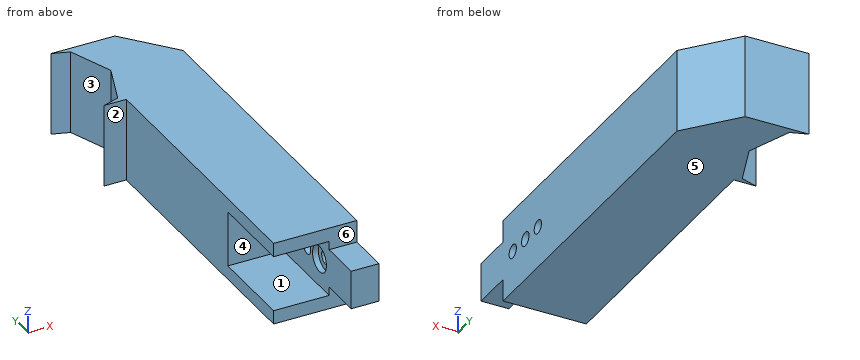
Autodesk Inventor part; units mm, degrees
ref_plane "YZ Plane" through (0, 0, 0) normal (1, 0, 0) x (0, 1, 0)
ref_plane "XZ Plane" through (0, 0, 0) normal (0, 1, 0) x (-1, 0, 0)
ref_plane "XY Plane" through (0, 0, 0) normal (0, 0, 1) x (1, 0, 0)
sketch "Sketch1" plane through (0, 0, 0) normal (0, 0, 1) x (1, 0, 0)
  line L0 (0, 0) -> (25, 0)
  line L1 (25, 0) -> (25, 40)
  line L2 (25, 40) -> (0, 40)
  line L3 (0, 40) -> (0, 0)
  dimension "d1" = 25
  dimension "d2" = 40
  dimension "d3" = 25
extrude "Extrusion1" add sketch "Sketch1" against normal blind 30
sketch "Sketch2" plane through (25, 0, 0) normal (1, 0, 0) x (0, 0, -1)
  line L0 (0, 0) -> (30, 0)
  circle A0 centre (15, 6.56) radius 2.46
extrude "Extrusion2" cut sketch "Sketch2" against normal blind 30
sketch "Sketch3" plane through (0, 0, 0) normal (-1, 0, 0) x (0, 0, 1)
  line L0 (0, 0) -> (-30, 0)
  line L1 (-25.05, 0) -> (-4.95, 0)
  line L2 (-4.95, 0) -> (-4.95, 33.12)
  line L3 (-4.95, 33.12) -> (-25.05, 33.12)
  line L4 (-25.05, 33.12) -> (-25.05, 0)
  dimension "d11" = 20.1
extrude "Extrusion3" cut sketch "Sketch3" against normal blind 20
sketch "Sketch4" plane through (0, 0, 0) normal (0, -1, 0) x (1, 0, 0)
  line L0 (20, -4.95) -> (20, -25.05)
  line L1 (20, -15) -> (25, -15)
  line L2 (25, 0) -> (25, -30)
  line L3 (20, -8.025) -> (25, -8.025)
  line L4 (25, -8.025) -> (25, -21.975)
  line L5 (25, -21.975) -> (20, -21.975)
  line L6 (20, -21.975) -> (20, -8.025)
  line L7 (20, -8.025) -> (25, -21.975) construction
  line L8 (25, -8.025) -> (20, -21.975) construction
  line L9 (25, -12.54) -> (25, -17.46)
  point P0 (0, 0)
  point P1 (22.5, -15)
  dimension "d14" = 13.95
extrude "Extrusion4" add sketch "Sketch4" along normal blind 15
sketch "Sketch5" plane through (20, 0, 0) normal (-1, 0, 0) x (0, 0, 1)
  circle A0 centre (-15, 6.56) radius 2.46
  circle A1 centre (-15, 6.56) radius 4.7025
  circle A2 centre (-15, 6.56) radius 2.46
  circle A3 centre (-15, 6.56) radius 2.46
  point P0 (0, 0)
  dimension "d17" = 9.405
extrude "Extrusion5" cut sketch "Sketch5" against normal blind 2.1
sketch "Sketch6" plane through (25, 0, 0) normal (1, 0, 0) x (0, 0, -1)
  circle A0 centre (15, 6.56) radius 4.7025
  line L0 (15, 6.56) -> (15, 23.56)
  circle A1 centre (15, 23.56) radius 2.46
  point P0 (0, 0)
  dimension "d20" = 17
  dimension "d21" = 4.92
extrude "Extrusion6" cut sketch "Sketch6" against normal blind 10 contours A1
sketch "Sketch7" plane through (20, 0, 0) normal (-1, 0, 0) x (0, 0, 1)
  circle A0 centre (-15, 23.56) radius 2.46
  circle A1 centre (-15, 23.56) radius 4.7025
  point P0 (0, 0)
  dimension "d24" = 9.405
extrude "Extrusion7" cut sketch "Sketch7" against normal blind 2.1
sketch "Sketch9" plane through (25, 0, 0) normal (1, 0, 0) x (0, 0, -1)
  circle A0 centre (15, 6.56) radius 2.46
  circle A1 centre (15, 6.56) radius 2.46
  circle A2 centre (15, 23.56) radius 2.46
  circle A3 centre (15, 23.56) radius 2.46
  line L0 (30, 40) -> (30, 0)
  line L1 (30, 0) -> (30, 40)
  line L2 (30, 40) -> (0, 40)
  line L3 (0, 40) -> (0, 0)
  line L4 (0, 0) -> (8.025, 0)
  line L5 (21.975, 0) -> (21.975, -15)
  line L6 (21.975, -15) -> (8.025, -15)
  line L7 (8.025, -15) -> (8.025, 0)
  line L8 (0, 0) -> (8.025, 0)
  line L9 (21.975, 0) -> (30, 0)
extrude "Extrusion8" add sketch "Sketch9" along normal blind 5
sketch "Sketch10" plane through (0, 40, 0) normal (0, 1, 0) x (1, 0, 0)
  line L0 (0, 30) -> (30, 30)
  line L1 (30, 0) -> (0, 0)
  line L2 (0, 30) -> (30, 30)
  line L3 (30, 30) -> (30, 0)
  line L4 (30, 0) -> (0, 0)
  line L5 (0, 0) -> (0, 30)
extrude "Extrusion9" add sketch "Sketch10" along normal blind 30
sketch "Sketch12" plane through (30, 0, 0) normal (1, 0, 0) x (0, 0, -1)
  circle A0 centre (15, 6.56) radius 2.46
  line L0 (15, 6.56) -> (15, 15.06)
  circle A1 centre (15, 15.06) radius 2.525
  point P0 (0, 0)
  dimension "d31" = 8.5
  dimension "d33" = 5.05
extrude "Extrusion10" cut sketch "Sketch12" against normal blind 30 contours A1
sketch "Sketch14" plane through (0, 0, 0) normal (0, 0, 1) x (1, 0, 0)
  line L0 (30, 70) -> (0, 70)
  line L1 (0, 100) -> (-8, 100)
  line L2 (30, 0) -> (30, 70)
  line L3 (30, 118) -> (30, 70)
  line L4 (30, 105) -> (30, 100)
  line L5 (-2, 134) -> (-8, 136)
  line L6 (-2, 134) -> (4, 118)
  line L7 (-2, 102) -> (-8, 100)
  line L8 (-2, 102) -> (4, 118)
  line L9 (0, 70) -> (30, 70)
  line L10 (0, 70) -> (0, 100)
  line L11 (15, 136) -> (30, 118)
  line L12 (-8, 136) -> (15, 136)
  point P0 (0, 0)
  dimension "d47" = 30
extrude "Extrusion12" add sketch "Sketch14" against normal blind 30
sketch "Sketch15" plane through (0, 0, -25.05) normal (-1, 0, 0) x (0, 0, 1)
  line L0 (0, 33.12) -> (20.1, 33.12)
  line L1 (20.1, 33.12) -> (20.1, 0)
  line L2 (0, 33.12) -> (20.1, 33.12)
  line L3 (20.1, 33.12) -> (20.1, 31.1)
  line L4 (20.1, 31.1) -> (0, 31.1)
  line L5 (0, 31.1) -> (0, 33.12)
  point P0 (25.05, 0)
  dimension "d57" = 2.02
extrude "Extrusion13" add sketch "Sketch15" against normal blind 20
properties part number "32mm_x_30mm"
Check sheet for the modelled part. Datum: model origin and axes. Units: mm. Face numbers are marked on the shaded views. A direction names the side the tool comes from. Round coordinates to 2 decimals unless told otherwise and drop trailing zeros. Order: outer loops, then holes, each group sorted by start corner. A loop starts at its lowest first (then second) coordinate and runs counter-clockwise, first axis right, second up. Notation, with made-up numbers: (44, 72.25) - (94, 72.25) arc R24 cw to (94, 86.25) - close; hole circle Ø7 at (79, 65.5). An arc over 180 degrees is marked (long way). Write item = value, one per line.
Q1. Go/stop test with flat-tipped pins: pin 1 (4 mm diameter, centred on x = 25, z = -24.5, fed in from +Y); pin 2 (10 mm diameter, centred on y = 81.5, z = -24.5, fed in from -X); pin 3 (4 mm diameter, centred on x = 16.5, z = -5.5, fed in from -Y). Record where each tip stops, or that it passes through.
Computed:
pin_1 = 126.4
pin_2 = 0
pin_3 = 0
Q2. Draft check along Z on the marked faces 4, 5 and 6. Enter one of: pulls with the +Z half, pulls with the -Z half, needs draft (parallel to the pull), parting line crosses it, or undercut.
Computed:
face_4 = undercut
face_5 = pulls with the -Z half
face_6 = needs draft
Q3. Section check D-D (x = 1.5). Record the boundary of the cut face in (y, z).
Computed:
outline = (0, -30) - (111.33, -30) - (111.33, 0) - (0, 0) - (0, -4.95) - (31.1, -4.95) - (31.1, -25.05) - (0, -25.05) - close; (124.67, -30) - (136, -30) - (136, 0) - (124.67, 0) - close
Q4. Section check B-B (x = 26). Record the boundary of the cut face in (y, z) (3 decimals).
Computed:
outline = (-15, -21.975) - (0, -21.975) - (0, -30) - (122.8, -30) - (122.8, 0) - (0, 0) - (0, -8.025) - (-15, -8.025) - close; hole circle Ø4.92 at (6.56, -15); hole circle Ø5.05 at (15.06, -15); hole circle Ø4.92 at (23.56, -15)
Q5. Thickness scan on line 1 along Z through (x, y) = (26, 6.56); line 2 along Y through (x, z) = (21.35, -15) (1 decimal); line 3 along Y through (x, z) = (25.25, -15) (3 decimals). Record the ranges inside material, lowest first.
Computed:
line_1 = -30 to -17.46, -12.54 to 0
line_2 = -15 to 1.9, 11.3 to 12.5, 17.6 to 18.9, 28.3 to 128.4
line_3 = -15 to 4.1, 9.02 to 12.535, 17.585 to 21.1, 26.02 to 123.7
Q6. Tool access check on the marked faces 1, 2 and 3. Record the directions out of +Z, -Z, +X, -X, +Y, -Y that give a thin tool (end or side, any length) a straight path to the whole face; none if there is none.
Computed:
face_1 = -X, -Y
face_2 = +Z, -Z, -X, -Y
face_3 = +Z, -Z, -X
Q7. Section check A-A (y = 15.06). Record the boundary of the cut face in (x, z) (3 decimals).
Computed:
outline = (0, -30) - (30, -30) - (30, -17.525) - (20, -17.525) - (20, -25.05) - (0, -25.05) - close; (0, -4.95) - (20, -4.95) - (20, -12.475) - (30, -12.475) - (30, 0) - (0, 0) - close
Q8. Section check C-C (z = -15). State how many separate pieces and enclosed holes the cut face has, and give its area (3 significant figures).
Computed:
separate_pieces = 4
enclosed_holes = 0
area = 3,290 mm^2
